```python
from build123d import *

# Parameters (mm, degrees)
SKETCH1_W           = 50.8
SKETCH1_H           = 127
SKETCH1_R           = 3.96875
SKETCH1_R_2         = 3.3734375
BOSS_EXTRUDE2_DEPTH = 12.7
CUT_EXTRUDE1_DEPTH  = 6.35
CUT_EXTRUDE2_START  = -12.7
SKETCH3_R           = 5.55625
CUT_EXTRUDE2_DEPTH  = 6.35
CUT_EXTRUDE3_START  = -12.7
SKETCH4_R           = 7.62
CUT_EXTRUDE3_DEPTH  = 6.35


with BuildPart() as part:
    # Sketch1 → Boss-Extrude2 (new body)
    with BuildSketch(Plane.XY):
        with Locations((25.4, 63.5)):
            Rectangle(SKETCH1_W, SKETCH1_H)
        with Locations((25.4, 12.7)):
            Circle(SKETCH1_R, mode=Mode.SUBTRACT)
        with Locations((25.4, 116.84)):
            Circle(SKETCH1_R_2, mode=Mode.SUBTRACT)
        with Locations((25.4, 91.44)):
            Circle(SKETCH1_R_2, mode=Mode.SUBTRACT)
        with BuildLine():
            ThreePointArc((42.2275, 51.256646253), (25.4, 54.76875), (8.5725, 51.256646253))
            ThreePointArc((8.5725, 51.256646253), (6.522580542, 46.031726796), (11.7475, 43.981807338))
            ThreePointArc((11.7475, 43.981807338), (25.4, 46.83125), (39.0525, 43.981807338))
            ThreePointArc((39.0525, 43.981807338), (44.277419458, 46.031726796), (42.2275, 51.256646253))
        make_face(mode=Mode.SUBTRACT)
    extrude(amount=BOSS_EXTRUDE2_DEPTH)

    # Sketch1<3> → Cut-Extrude1 (cut)
    with BuildSketch(Plane.XY):
        with BuildLine():
            ThreePointArc((37.5285, 40.489884658), (25.4, 43.02125), (13.2715, 40.489884658))
            ThreePointArc((13.2715, 40.489884658), (3.030657863, 44.507726796), (7.0485, 54.748568933))
            ThreePointArc((7.0485, 54.748568933), (25.4, 58.57875), (43.7515, 54.748568933))
            ThreePointArc((43.7515, 54.748568933), (47.769342137, 44.507726796), (37.5285, 40.489884658))
        make_face()
        with BuildLine():
            ThreePointArc((39.0525, 43.981807338), (44.277419458, 46.031726796), (42.2275, 51.256646253))
            ThreePointArc((42.2275, 51.256646253), (25.4, 54.76875), (8.5725, 51.256646253))
            ThreePointArc((8.5725, 51.256646253), (6.522580542, 46.031726796), (11.7475, 43.981807338))
            ThreePointArc((11.7475, 43.981807338), (25.4, 46.83125), (39.0525, 43.981807338))
        make_face(mode=Mode.SUBTRACT)
    extrude(amount=CUT_EXTRUDE1_DEPTH, mode=Mode.SUBTRACT)

    # Sketch3 → Cut-Extrude2 (cut)
    with BuildSketch(Plane(origin=(0, 0, 0), x_dir=(-1, 0, 0), z_dir=(0, 0, -1)).offset(CUT_EXTRUDE2_START)):
        with Locations(Location((-25.4, 116.84, 0), (0, 0, 180))):
            Circle(SKETCH3_R)
        with Locations(Location((-25.4, 91.44, 0), (0, 0, 180))):
            Circle(SKETCH3_R)
    extrude(amount=CUT_EXTRUDE2_DEPTH, mode=Mode.SUBTRACT)

    # Sketch4 → Cut-Extrude3 (cut)
    with BuildSketch(Plane.XY.offset(12.7).offset(CUT_EXTRUDE3_START)):
        with Locations((25.4, 12.7)):
            Circle(SKETCH4_R)
    extrude(amount=CUT_EXTRUDE3_DEPTH, mode=Mode.SUBTRACT)


solid = part.part
```
Can you work these out from the model? Positions are in its coordinate system, mm. A direction names the side the tool comes from. Coordinates: 2 decimals unless noted, no trailing zeros. Loops run counter-clockwise (first coordinate to the right, second up) from the corner with the lowest first, then second, coordinate; pieces in that order, holes last. Notation, with made-up numbers: (-5, -10.75) -> (26, -10.75) arc R9 ccw to (26, -4.75) -> close; hole circle Ø2 at (-30, 79). An arc over 180 degrees is marked (long way). Put each result on its own line as item: value. Start each with the question number.
Q1. Thinking about a two-plate mould opening in X: for faces 4 (the face through (0, 63, 6)), 5 (the face through (25.64, 54.77, 9.48)), 6 (the face through (25, 0, 6)), which applies, pulls with the +X half, pulls with the -X half, needs draft (parallel to the pull), parting line crosses it, or undercut?
Q2. I want a section at D-D (z = 4). Write out the boundary of the cut face in (x, y).
Q3. I want a section at B-B (z = 10.25). Write out the boundary of the cut face in (x, y), plus the area to 3 significant figures.
Q4. If I drill on line 1 (X direction, y = 116.84, z = 4.25); line 2 (X direction, y = 117, z = 7.25); line 3 (Y direction, x = 22, z = 9.5), over which ranges is the centre line in solid material (lowest first)? Write a range as [from, to].
Q5. I'm going to push flat-ended pins straight in: P1, Ø4.5, axis at x = 23, y = 16, coming from the -Z side; P2, Ø3.5, axis at x = 24.5, y = 118.5, coming from the +Z side. Where does each tip first touch, or does it pass through?
Q6. For faces 1 (the face through (21.435, 12.874, 9.481)), 2 (the face through (24.68, 85.93, 9.57)), 3 (the face through (47.84, 44.67, 3.13)), which set-ups out of +Z, -Z, +X, -X, +Y, -Y let a thin tool reach every point of the face, with its end or its side?
Q7. I want a section at A-A (y = 91.44). Write out the boundary of the cut face in (x, z).
Q8. I want a section at C-C (x = 10). Write out the boundary of the cut face in (y, z).
Taken from the geometry:
1. face 4: pulls with the -X half
1. face 5: undercut
1. face 6: needs draft
2. outline: (0, 0) -> (50.8, 0) -> (50.8, 127) -> (0, 127) -> close; hole (7.05, 54.75) arc R7.78 ccw to (13.27, 40.49) arc R30.32 cw to (37.53, 40.49) arc R7.78 ccw to (43.75, 54.75) arc R45.88 ccw to start; hole circle Ø15.24 at (25.4, 12.7); hole circle Ø6.75 at (25.4, 91.44); hole circle Ø6.75 at (25.4, 116.84)
3. outline: (0, 0) -> (50.8, 0) -> (50.8, 127) -> (0, 127) -> close; hole (8.57, 51.26) arc R3.97 ccw to (11.75, 43.98) arc R34.13 cw to (39.05, 43.98) arc R3.97 ccw to (42.23, 51.26) arc R42.07 ccw to start; hole circle Ø11.11 at (25.4, 91.44); hole circle Ø11.11 at (25.4, 116.84); hole circle Ø7.94 at (25.4, 12.7)
3. area: 5,910 mm2
4. line 1: x = [0, 22.03], [28.77, 50.8]
4. line 2: x = [0, 19.85], [30.95, 50.8]
4. line 3: y = [0, 10.65], [14.75, 46.66], [54.63, 87.05], [95.83, 112.45], [121.23, 127]
5. P1: stops at z = 6.35
5. P2: stops at z = 6.35
6. face 1: +Z, -Z
6. face 2: +Z
6. face 3: -Z
7. outline: (0, 0) -> (22.03, 0) -> (22.03, 6.35) -> (19.84, 6.35) -> (19.84, 12.7) -> (0, 12.7) -> close; (28.77, 0) -> (50.8, 0) -> (50.8, 12.7) -> (30.96, 12.7) -> (30.96, 6.35) -> (28.77, 6.35) -> close
8. outline: (0, 0) -> (39.84, 0) -> (39.84, 6.35) -> (43.65, 6.35) -> (43.65, 12.7) -> (0, 12.7) -> close; (51.85, 6.35) -> (55.92, 6.35) -> (55.92, 0) -> (127, 0) -> (127, 12.7) -> (51.85, 12.7) -> close
